Build history of the part. All positions in model axes, mm. A direction names the side the tool comes from. Round coordinates to 2 decimals unless told otherwise and drop trailing zeros. Write each loop counter-clockwise with the first axis right and the second up, starting at its lowest first coordinate (ties: lowest second). Pieces come first, ordered by that corner, then holes. Notation, with made-up numbers: (-27, 47.25) -> (21, 47.25) arc R7 cw to (21, 60.25) -> close; hole circle Ø9 at (67.5, 29.5). An arc over 180 degrees is marked (long way). Return JSON: item names as keys, results as strings.
from build123d import *

# Parameters (mm, degrees)
SKETCH1_R           = 1.5
BOSS_EXTRUDE1_DEPTH = 9.05
SKETCH2_W           = 4
SKETCH2_H           = 3
BOSS_EXTRUDE2_DEPTH = 2
SKETCH3_W           = 4
SKETCH3_H           = 3
BOSS_EXTRUDE3_DEPTH = 2


with BuildPart() as part:
    # Sketch1 → Boss-Extrude1 (new body, symmetric)
    with BuildSketch(Plane.XY):
        Circle(SKETCH1_R)
    extrude(amount=BOSS_EXTRUDE1_DEPTH, both=True)

    # Sketch2 → Boss-Extrude2 (add)
    with BuildSketch(Plane.XY.offset(9.05)):
        Rectangle(SKETCH2_W, SKETCH2_H)
    extrude(amount=BOSS_EXTRUDE2_DEPTH)

    # Sketch3 → Boss-Extrude3 (add)
    with BuildSketch(Plane(origin=(0, 0, -9.05), x_dir=(-1, 0, 0), z_dir=(0, 0, -1))):
        Rectangle(SKETCH3_W, SKETCH3_H)
    extrude(amount=BOSS_EXTRUDE3_DEPTH)


solid = part.part
Q1. Saw through at A-A on y = 0. List the corners of the cut face in (x, z), then the cut area to 3 significant figures.
Verdict:
{"outline": "(-2, -11.05) -> (2, -11.05) -> (2, -9.05) -> (1.5, -9.05) -> (1.5, 9.05) -> (2, 9.05) -> (2, 11.05) -> (-2, 11.05) -> (-2, 9.05) -> (-1.5, 9.05) -> (-1.5, -9.05) -> (-2, -9.05) -> close", "area": "70.3 mm²"}
Q2. Saw through at C-C on z = 5.5. List the corners of the cut face in (x, y).
Verdict:
{"outline": "circle Ø3 at (0, 0)"}
Q3. Wall check: L1, parallel to Z at x = -1.3, y = -1; L2, parallel to X at y = 0.1, z = 7.5. Give the ranges that are in metal, low to high.
Verdict:
{"L1": "z = -11.05 to -9.05, 9.05 to 11.05", "L2": "x = -1.5 to 1.5"}
Q4. 3-axis set-ups, long thin cutter, end or side, ignore diameter. For faces 1 (the flat face through (-2, 0, 10)), 2 (the cylindrical face through (-1.5, 0.07, 0.13)), 3 (the flat face through (-1.7, 0, 9.05)), 4 (the flat face through (1.7, 0, -9.05)), 5 (the flat face through (0, 1.5, -10)): which of +Z, -Z, +X, -X, +Y, -Y reach the whole face in a straight line?
Verdict:
{"face 1": "+Z, -Z, -X, +Y, -Y", "face 2": "none", "face 3": "-X", "face 4": "+X", "face 5": "+Z, -Z, +X, -X, +Y"}
Q5. Pin check, flat tip, straight feed: pin 1 Ø1.5 at (x, z) = (1.5, 0.5) entering from +Y. Stop position of the tip, or through.
Verdict:
{"pin 1": "stops at y = 1.3"}
Q6. Saw through at B-B on x = 1.25. List the corners of the cut face in (y, z), then the cut area to 3 significant figures.
Verdict:
{"outline": "(-1.5, -11.05) -> (1.5, -11.05) -> (1.5, -9.05) -> (0.83, -9.05) -> (0.83, 9.05) -> (1.5, 9.05) -> (1.5, 11.05) -> (-1.5, 11.05) -> (-1.5, 9.05) -> (-0.83, 9.05) -> (-0.83, -9.05) -> (-1.5, -9.05) -> close", "area": "42.0 mm²"}
